Autodesk Inventor part; units mm, degrees
ref_plane "YZ Plane" through (0, 0, 0) normal (1, 0, 0) x (0, 1, 0)
ref_plane "XZ Plane" through (0, 0, 0) normal (0, 1, 0) x (-1, 0, 0)
ref_plane "XY Plane" through (0, 0, 0) normal (0, 0, 1) x (1, 0, 0)
sketch "Sketch1" plane through (0, 0, 0) normal (0, 1, 0) x (-1, 0, 0)
  line L0 (64.8, -22.3) -> (-64.8, -22.3)
  line L1 (-64.8, -22.3) -> (-64.8, 22.3)
  line L2 (-64.8, 22.3) -> (64.8, 22.3)
  line L3 (64.8, 22.3) -> (64.8, -22.3)
  point P0 (0, 0)
  point P1 (64.8, 0)
  point P2 (0, -22.3)
  dimension "d0" = 129.6
  dimension "d1" = 44.6
extrude "Extrusion1" add sketch "Sketch1" along normal blind 3
sketch "Sketch2" plane through (0, 3, 0) normal (0, 1, 0) x (1, 0, 0)
  line L0 (-64.8, -22.3) -> (64.8, -22.3) construction
  line L1 (64.8, -22.3) -> (64.8, 22.3) construction
  line L2 (64.8, 22.3) -> (-64.8, 22.3) construction
  line L3 (-64.8, 22.3) -> (-64.8, -22.3) construction
  line L4 (-40, 18.55) -> (40, 18.55) construction
  line L5 (40, 18.55) -> (40, -17.45) construction
  line L6 (40, -17.45) -> (-40, -17.45) construction
  line L7 (-40, -17.45) -> (-40, 18.55) construction
  circle A0 centre (-37.5, 16.05) radius 1.25 construction
  circle A1 centre (37.5, 16.05) radius 1.25 construction
  circle A2 centre (37.5, -14.95) radius 1.25 construction
  circle A3 centre (-37.5, -14.95) radius 1.25 construction
  line L8 (-37.5, 12.5) -> (37.5, 12.5) construction
  line L9 (37.5, 12.5) -> (37.5, -12.5) construction
  line L10 (37.5, -12.5) -> (-37.5, -12.5) construction
  line L11 (-37.5, -12.5) -> (-37.5, 12.5) construction
  line L12 (-40, 18.55) -> (-35, 18.55)
  line L13 (-35, 18.55) -> (-35, 13.55)
  line L14 (-35, 13.55) -> (-40, 13.55)
  line L15 (-40, 13.55) -> (-40, 18.55)
  line L16 (-40, 18.55) -> (-35, 13.55) construction
  line L17 (-35, 18.55) -> (-40, 13.55) construction
  line L18 (35, 18.55) -> (40, 18.55)
  line L19 (40, 18.55) -> (40, 13.55)
  line L20 (40, 13.55) -> (35, 13.55)
  line L21 (35, 13.55) -> (35, 18.55)
  line L22 (35, 18.55) -> (40, 13.55) construction
  line L23 (40, 18.55) -> (35, 13.55) construction
  line L24 (35, -12.45) -> (40, -12.45)
  line L25 (40, -12.45) -> (40, -17.45)
  line L26 (40, -17.45) -> (35, -17.45)
  line L27 (35, -17.45) -> (35, -12.45)
  line L28 (35, -12.45) -> (40, -17.45) construction
  line L29 (40, -12.45) -> (35, -17.45) construction
  line L30 (-40, -12.45) -> (-35, -12.45)
  line L31 (-35, -12.45) -> (-35, -17.45)
  line L32 (-35, -17.45) -> (-40, -17.45)
  line L33 (-40, -17.45) -> (-40, -12.45)
  line L34 (-40, -12.45) -> (-35, -17.45) construction
  line L35 (-35, -12.45) -> (-40, -17.45) construction
  point P0 (0, 0)
  point P1 (0, 12.5)
  point P2 (0, 22.3)
  dimension "d4" = 80
  dimension "d5" = 36
  dimension "d6" = 2.5
  dimension "d7" = 2.5
  dimension "d8" = 2.5
  dimension "d9" = 2.5
  dimension "d10" = 2.5
  dimension "d12" = 75
  dimension "d13" = 25
  dimension "d14" = 2.5
  dimension "d15" = 4.95
  dimension "d16" = 9.8
  dimension "d17" = 5
extrude "Extrusion2" add sketch "Sketch2" along normal blind 3
sketch "Sketch3" plane through (0, 6, 0) normal (0, 1, 0) x (1, 0, 0)
  line L0 (-35, 18.55) -> (-40, 13.55) construction
  point P0 (0, 0)
  point P1 (-37.5, -14.95)
  point P2 (-37.5, 16.05)
  point P3 (37.5, 16.05)
  point P4 (37.5, -14.95)
hole "Hole1" at (-37.5, 6, 14.95) at (-37.5, 6, -16.05) at (37.5, 6, -16.05) at (37.5, 6, 14.95) direction (0, -1, 0) diameter 3.5 depth 4
chamfer "Chamfer1" distance 3 angle 45 16 edges at (-37.5, 3, -13.55) (-40, 3, -16.05) (-37.5, 3, -18.55) (-35, 3, -16.05) (-37.5, 3, 12.45) (-40, 3, 14.95) (-37.5, 3, 17.45) (-35, 3, 14.95) (37.5, 3, -13.55) (35, 3, -16.05) (37.5, 3, -18.55) (40, 3, -16.05) (37.5, 3, 12.45) (35, 3, 14.95) (37.5, 3, 17.45) (40, 3, 14.95)
sketch "Sketch4" plane through (0, 3, 0) normal (0, 1, 0) x (1, 0, 0)
  line L0 (43, 10.55) -> (43, 21.55) construction
  line L1 (32, 10.55) -> (43, 10.55) construction
  line L2 (32, 21.55) -> (32, 10.55) construction
  line L3 (43, 21.55) -> (32, 21.55) construction
  line L4 (-32, 10.55) -> (-32, 21.55) construction
  line L5 (-43, 10.55) -> (-32, 10.55) construction
  line L6 (-43, 21.55) -> (-43, 10.55) construction
  line L7 (-32, 21.55) -> (-43, 21.55) construction
  line L8 (-64.8, -22.3) -> (64.8, -22.3) construction
  line L9 (64.8, -22.3) -> (64.8, 22.3) construction
  line L10 (64.8, 22.3) -> (-64.8, 22.3) construction
  line L11 (-64.8, 22.3) -> (-64.8, -22.3) construction
  line L12 (-43, -9.45) -> (-43, -20.45) construction
  line L13 (-32, -9.45) -> (-43, -9.45) construction
  line L14 (-32, -20.45) -> (-32, -9.45) construction
  line L15 (-43, -20.45) -> (-32, -20.45) construction
  line L16 (32, -9.45) -> (32, -20.45) construction
  line L17 (43, -9.45) -> (32, -9.45) construction
  line L18 (43, -20.45) -> (43, -9.45) construction
  line L19 (32, -20.45) -> (43, -20.45) construction
  line L20 (64.8, 22.3) -> (-64.8, 22.3) construction
  line L21 (-31, 22.3) -> (-29, 20.3)
  line L22 (-29, 20.3) -> (-9, 20.3)
  line L23 (-9, 20.3) -> (-7, 22.3)
  line L24 (-31, 22.3) -> (-7, 22.3)
  point P0 (0, 0)
  dimension "d31" = 2
  dimension "d32" = 20
  dimension "d33" = 135
  dimension "d34" = 135
  dimension "d35" = 1
extrude "Extrusion3" cut sketch "Sketch4" against normal blind 3
chamfer "Chamfer2" distance 3 angle 45 4 edges at (-64.8, 1.5, -22.3) (-64.8, 1.5, 22.3) (64.8, 1.5, 22.3) (64.8, 1.5, -22.3)
sketch "Sketch5" plane through (0, 3, 0) normal (0, 1, 0) x (1, 0, 0)
  line L0 (43, 10.55) -> (43, 21.55) construction
  line L1 (32, 10.55) -> (43, 10.55) construction
  line L2 (32, 21.55) -> (32, 10.55) construction
  line L3 (43, 21.55) -> (32, 21.55) construction
  line L4 (-32, 10.55) -> (-32, 21.55) construction
  line L5 (-43, 10.55) -> (-32, 10.55) construction
  line L6 (-43, 21.55) -> (-43, 10.55) construction
  line L7 (-32, 21.55) -> (-43, 21.55) construction
  line L8 (-43, -9.45) -> (-43, -20.45) construction
  line L9 (-32, -9.45) -> (-43, -9.45) construction
  line L10 (-32, -20.45) -> (-32, -9.45) construction
  line L11 (-43, -20.45) -> (-32, -20.45) construction
  line L12 (32, -9.45) -> (32, -20.45) construction
  line L13 (43, -9.45) -> (32, -9.45) construction
  line L14 (43, -20.45) -> (43, -9.45) construction
  line L15 (32, -20.45) -> (43, -20.45) construction
  line L16 (61.8, 22.3) -> (64.8, 19.3) construction
  line L17 (61.8, 22.3) -> (-7, 22.3) construction
  line L18 (-7, 22.3) -> (-9, 20.3) construction
  line L19 (-9, 20.3) -> (-29, 20.3) construction
  line L20 (-29, 20.3) -> (-31, 22.3) construction
  line L21 (-31, 22.3) -> (-61.8, 22.3) construction
  line L22 (-64.8, 19.3) -> (-61.8, 22.3) construction
  line L23 (-64.8, 19.3) -> (-64.8, -19.3) construction
  line L24 (-61.8, -22.3) -> (-64.8, -19.3) construction
  line L25 (-61.8, -22.3) -> (61.8, -22.3) construction
  line L26 (64.8, -19.3) -> (61.8, -22.3) construction
  line L27 (64.8, -19.3) -> (64.8, 19.3) construction
  point P0 (0, 0)
  point P1 (-60, 17.5)
  point P2 (-60, -17.5)
  point P3 (60, -17.5)
  point P4 (60, 17.5)
  dimension "d49" = 4.8
  dimension "d50" = 4.8
  dimension "d51" = 4.8
  dimension "d52" = 4.8
hole "Hole2" at (-60, 3, -17.5) at (-60, 3, 17.5) at (60, 3, 17.5) at (60, 3, -17.5) direction (0, -1, 0) diameter 3.4 depth 4
equation "\"d8\" = d7"
equation "\"d9\" = d7"
equation "\"d10\" = d7"
equation "\"d34\" = d33"
properties part number "VFD_Mount"
Design review of the part built by this model. Coordinates are the model's own, in mm. A direction names the side the tool comes from. Coordinates: 2 decimals unless noted, no trailing zeros. Order: outer loops, then holes, each group sorted by start corner. A loop starts at its lowest first (then second) coordinate and runs counter-clockwise, first axis right, second up. Notation, with made-up numbers: (88, 68) -> (95, 68) arc R23 ccw to (95, 88) -> close; hole circle Ø4 at (21, 44.25). An arc over 180 degrees is marked (long way). One line per item, written item: value. Start each with the question number.
Q1. Mouldability with a two-part tool opening along X and no side actions: class faces 6 (the flat face through (42, 4, 15)), 7 (the flat face through (-38, 2, 15)), 8 (the flat face through (37.58, 4.19, 19.26)) as pulls with the +X half, pulls with the -X half, needs draft (parallel to the pull), parting line crosses it, or undercut.
Q2. For probe 1 along Z at (x, y) = (-60, 1.1); probe 2 along X at (y, z) = (0.95, -17.5); probe 3 along Y at (x, z) = (30, 6), list the stretches that pass through material, from the lowest coordinate up.
Q3. Insertion check: pin 1 Ø4.5 at (x, z) = (-60, -17.5) entering from +Y; pin 2 Ø1 at (x, z) = (36.5, -16) entering from +Y; pin 3 Ø1.5 at (x, y) = (-17.5, 2) entering from -Z; pin 4 Ø2.5 at (x, z) = (60, 17.5) entering from +Y. Each pin has a flat end and moves straight along its axis. Give the tip position at first contact, or say it passes through.
Q4. Take a section at A-A, the plane x = -60. State the section outline as (y, z) points, then the cut area to 3 significant figures.
Q5. Take a section at D-D, the plane x = -1. State the section outline as (y, z) points, then the cut area to 3 significant figures.
Q6. Take a section at C-C, the plane z = -6.5. State the section outline as (x, y) points, then the cut area to 3 significant figures.
Q7. Tool access review of faces 1 (the flat face through (37, 2, -16)), 2 (the flat face through (-19, 2, -20.3)), 3 (the flat face through (-63.3, 1.5, 20.8)), 4 (the flat face through (-33, 4, 15)), 5 (the flat face through (63.3, 1.5, -20.8)): name each direction out of +Z, -Z, +X, -X, +Y, -Y from which nothing blocks a thin tool from reaching the whole face with its end or side.
Values follow:
1. face 6: pulls with the +X half
1. face 7: undercut
1. face 8: needs draft
2. probe 1: z = -22.3 to -19.2, -15.8 to 15.8, 19.2 to 22.3
2. probe 2: x = -64.8 to -61.7, -58.3 to 58.3, 61.7 to 64.8
2. probe 3: y = 0 to 3
3. pin 1: stops at y = 3
3. pin 2: stops at y = 2
3. pin 3: stops at z = -20.3
3. pin 4: passes through
4. outline: (0, -22.3) -> (3, -22.3) -> (3, -19.2) -> (0, -19.2) -> close; (0, -15.8) -> (3, -15.8) -> (3, 15.8) -> (0, 15.8) -> close; (0, 19.2) -> (3, 19.2) -> (3, 22.3) -> (0, 22.3) -> close
4. area: 113 mm2
5. outline: (0, -22.3) -> (3, -22.3) -> (3, 22.3) -> (0, 22.3) -> close
5. area: 134 mm2
6. outline: (-64.8, 0) -> (64.8, 0) -> (64.8, 3) -> (-64.8, 3) -> close
6. area: 389 mm2
7. face 1: +Y
7. face 2: -Z, +Y, -Y
7. face 3: +Z, -X, +Y, -Y
7. face 4: +Z, -Z, +Y
7. face 5: -Z, +X, +Y, -Y
